Can you work these out from the drawing? Everything is in mm from the part's minimum corner. Give positions to 0.01 mm unless a question says otherwise; leave off trailing zeros. Loops run counter-clockwise (first coordinate to the right, second up) from the corner with the lowest first, then second, coordinate; pieces in that order, holes last.
Q1. Will these pins go through, and if not, where does the flat tip stop? P1, Ø8, axis at x = 42.5, z = 50.5, coming from the +Y side; P2, Ø2, axis at x = 36.5, y = 4, coming from the -Z side; P3, Ø1, axis at y = 3, z = 67, coming from the -X side.
Q2. If we section it at B-B (z = 45.72): Please give me the cut outline in (x, y).
Q3. We'd pull the mould along X, two halves only. Please class the marked faces 1 and 2: +X half, -X half, draft (parallel to the pull), parting line (faces both ways), or undercut.
Q4. I need wall thicknesses on line 1 (X direction, y = 0.45, z = 45.72); line 2 (X direction, y = 1.2, z = 47.5); line 3 (Z direction, x = 37.5, y = 3.5). Which ranges of each line are inside material? Lowest first, please.
Q5. If we section it at A-A (x = 45.72): Please give me the cut outline in (y, z), plus the area to 3 significant figures.
Q6. If we section it at C-C (y = 2.15): Please give me the cut outline in (x, z).
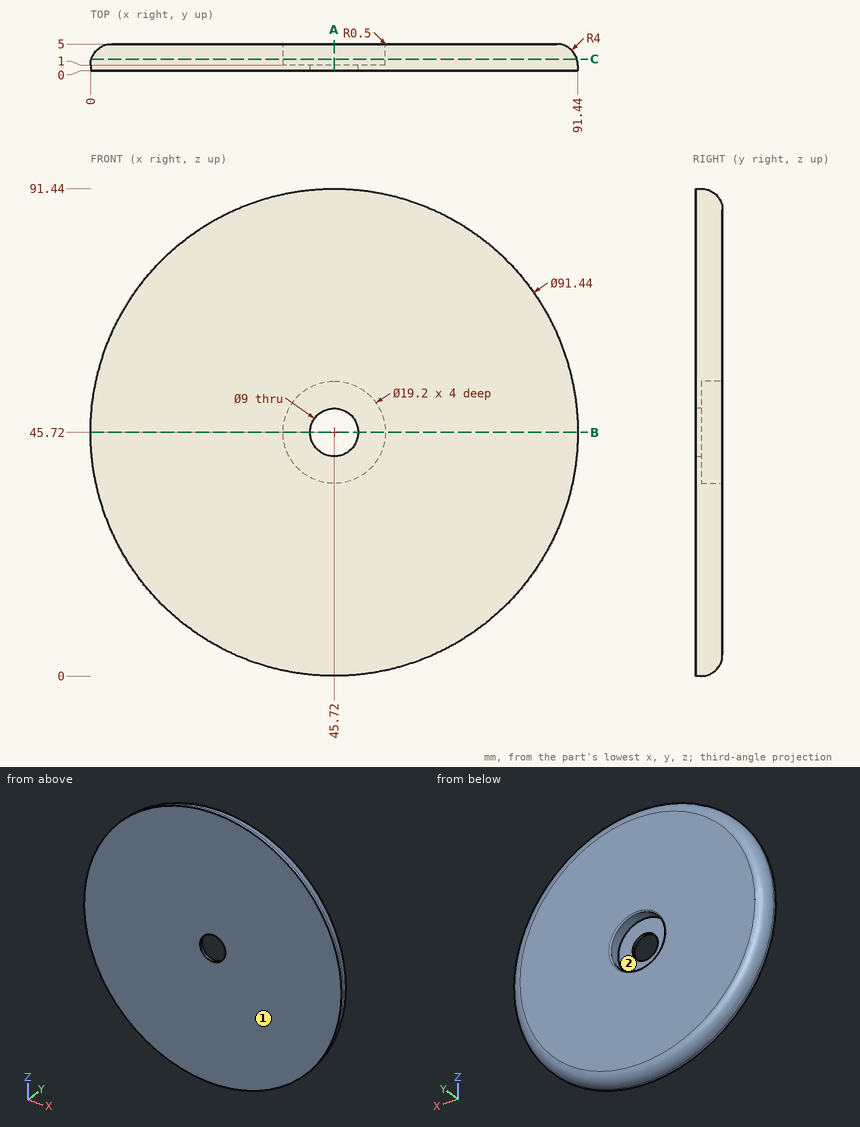
Check sheet entries:
1. P1: stops at y = 4.87
1. P2: stops at z = 1.45
1. P3: stops at x = 5.47
2. outline: (0, 0) - (41.22, 0) - (41.22, 1) - (36.12, 1) - (36.12, 4.5) arc R0.5 ccw to (35.62, 5) - (4, 5) arc R4 ccw to (0, 1) - close; (50.22, 0) - (91.44, 0) - (91.44, 1) arc R4 ccw to (87.44, 5) - (55.82, 5) arc R0.5 ccw to (55.32, 4.5) - (55.32, 1) - (50.22, 1) - close
3. face 1: draft
3. face 2: undercut
4. line 1: x = 0 to 41.22, 50.22 to 91.44
4. line 2: x = 0.04 to 36.29, 55.15 to 91.4
4. line 3: z = 1.64 to 40.76, 50.68 to 89.8
5. outline: (0, 0) - (1, 0) arc R4 ccw to (5, 4) - (5, 35.62) arc R0.5 ccw to (4.5, 36.12) - (1, 36.12) - (1, 41.22) - (0, 41.22) - close; (0, 50.22) - (1, 50.22) - (1, 55.32) - (4.5, 55.32) arc R0.5 ccw to (5, 55.82) - (5, 87.44) arc R4 ccw to (1, 91.44) - (0, 91.44) - close
5. area: 364 mm2
6. outline: circle Ø91.1 at (45.72, 45.72); hole circle Ø19.2 at (45.72, 45.72)
